Could you check a few things on this model? Use its own coordinates, in mm. A direction names the side the tool comes from. Coordinates: 2 decimals unless noted, no trailing zeros. Write each loop counter-clockwise with the first axis right and the second up, starting at its lowest first coordinate (ties: lowest second). Pieces come first, ordered by that corner, then holes.
Autodesk Inventor part; units mm, degrees
ref_plane "Work Plane1" through (0, 15, 0) normal (0, 1, 0) x (-1, 0, 0)
ref_plane "YZ Plane" through (0, 0, 0) normal (1, 0, 0) x (0, 1, 0)
ref_plane "XY Plane" through (0, 0, 0) normal (0, 0, 1) x (1, 0, 0)
sketch "Sketch1" plane through (0, 0, 0) normal (0, 0, 1) x (1, 0, 0)
  line L0 (37.75, -20.25) -> (-37.75, -20.25)
  line L1 (-37.75, -20.25) -> (-37.75, 20.25)
  line L2 (-37.75, 20.25) -> (37.75, 20.25)
  line L3 (37.75, 20.25) -> (37.75, -20.25)
  point P0 (0, 0)
  point P1 (0, 20.25)
  point P2 (37.75, 0)
  dimension "d0" = 40.5
  dimension "d1" = 75.5
extrude "Extrusion1" add sketch "Sketch1" along normal blind 3
sketch "Sketch2" plane through (-37.75, 20.25, 0) normal (0, 1, 0) x (1, 0, 0)
  point P0 (37.75, 0)
ref_plane "Work Plane1" through (0, 15, 0) normal (0, 1, 0) x (-1, 0, 0)
sketch "Sketch3" plane through (0, 15, 0) normal (0, 1, 0) x (-1, 0, 0)
  line L0 (-37.75, 3) -> (37.75, 3)
  line L1 (7.25, 3) -> (-7.25, 3)
  line L2 (-7.25, 3) -> (-7.25, 6)
  line L3 (-7.25, 6) -> (7.25, 6)
  line L4 (7.25, 6) -> (7.25, 3)
  line L5 (7.25, 3) -> (-7.25, 3)
  point P0 (0, 6)
  point P1 (0, 3)
  dimension "d20" = 14.5
  dimension "d21" = 3
extrude "Extrusion2" add sketch "Sketch3" along normal blind 10
sketch "Sketch4" plane through (0, 0, 3) normal (0, 0, 1) x (1, 0, 0)
  line L0 (-30, -7) -> (-5, -7)
  line L1 (-5, -7) -> (-5, -13)
  line L2 (-5, -13) -> (-30, -13)
  line L3 (-30, -13) -> (-30, -7)
  line L4 (37.75, 20.25) -> (-37.75, 20.25)
  line L5 (0, 20.25) -> (0, -20.25) construction
  line L6 (-37.75, -20.25) -> (37.75, -20.25)
  line L7 (30, -7) -> (5, -7)
  line L8 (5, -7) -> (5, -13)
  line L9 (5, -13) -> (30, -13)
  line L10 (30, -13) -> (30, -7)
  point P0 (0, 0)
  point P1 (-5, -10)
  point P2 (-17.5, -7)
  point P3 (7.25, 20.25)
  point P4 (-7.25, 20.25)
  point P5 (0, 0)
  dimension "d9" = 25
  dimension "d10" = 6
  dimension "d11" = 5
  dimension "d12" = 7
extrude "Extrusion3" add sketch "Sketch4" along normal blind 5
sketch "Sketch5" plane through (-30, -13, 3) normal (0, -1, 0) x (1, 0, 0)
  line L0 (25, 0) -> (0, 0)
  line L1 (5, 0) -> (20, 0)
  line L2 (20, 0) -> (20, 3.5)
  line L3 (20, 3.5) -> (5, 3.5)
  line L4 (5, 3.5) -> (5, 0)
  line L5 (35, 5) -> (60, 5)
  line L6 (0, 0) -> (0, 5)
  line L7 (0, 5) -> (25, 5)
  line L8 (30, -3) -> (30, 5) construction
  line L9 (55, 0) -> (40, 0)
  line L10 (40, 0) -> (40, 3.5)
  line L11 (40, 3.5) -> (55, 3.5)
  line L12 (55, 3.5) -> (55, 0)
  point P0 (47.5, 5)
  point P1 (0, 2.5)
  point P2 (12.5, 3.5)
  point P3 (12.5, 5)
  point P4 (47.5, 3.5)
  point P5 (20, 0)
  dimension "d15" = 15
  dimension "d16" = 3.5
extrude "Extrusion4" cut sketch "Sketch5" against normal blind 3
properties part number "Pomodoro Robot Torso's back"
1. If we mould it in two halves opening along X, with no side actions, what happens to faces 6 (the face through (0, 25, 5)), 7 (the face through (5, -10, 5)), 8 (the face through (-30, -10, 5))? For each: pulls with the +X half, pulls with the -X half, needs draft (parallel to the pull), parting line crosses it, or undercut.
Verdict:
face 6: needs draft
face 7: undercut
face 8: pulls with the -X half
2. On a 3-axis mill with a long thin cutter (end or side, diameter ignored), from which of +Z, -Z, +X, -X, +Y, -Y can I reach the whole of each face in a straight line? I mean faces 1 (the face through (30, -10, 5)), 2 (the face through (-17, -13, 7)), 3 (the face through (-5, -10, 5)), 4 (the face through (17, -10, 5)), 5 (the face through (0, 15, 5)). Say none if no direction works.
Verdict:
face 1: +Z, +X, +Y, -Y
face 2: +Z, +X, -X, -Y
face 3: +Z, -Y
face 4: -Y
face 5: +Z, +X, -X
3. I want a section at B-B on x = 14.5. Please give me the cut outline in (y, z), plus the area to 3 significant figures.
Verdict:
outline: (-20.25, 0) - (20.25, 0) - (20.25, 3) - (-7, 3) - (-7, 8) - (-13, 8) - (-13, 6.5) - (-10, 6.5) - (-10, 3) - (-20.25, 3) - close
area: 141 mm2
4. I want a section at C-C on z = 2. Please give me the cut outline in (x, y), plus the area to 3 significant figures.
Verdict:
outline: (-37.75, -20.25) - (37.75, -20.25) - (37.75, 20.25) - (-37.75, 20.25) - close
area: 3,060 mm2
5. For pin 1 (1 mm diameter, centred on x = 18.5, z = 4.5, fed in from -Y); pin 2 (2.5 mm diameter, centred on x = -15, z = 6, fed in from +Y); pin 3 (3.5 mm diameter, centred on x = -4.5, z = 1, fed in from +Y), each with a flat end and sliding along its axis, tell me the tip position at first contact or that it passes through.
Verdict:
pin 1: stops at y = -10
pin 2: stops at y = -7
pin 3: stops at y = 20.25
6. I want a section at D-D on y = 21.5. Please give me the cut outline in (x, z), plus the area to 3 significant figures.
Verdict:
outline: (-7.25, 3) - (7.25, 3) - (7.25, 6) - (-7.25, 6) - close
area: 43.5 mm2
7. I want a section at A-A on y = -12. Please give me the cut outline in (x, z).
Verdict:
outline: (-37.75, 0) - (37.75, 0) - (37.75, 3) - (30, 3) - (30, 8) - (5, 8) - (5, 3) - (-5, 3) - (-5, 8) - (-30, 8) - (-30, 3) - (-37.75, 3) - close; hole (-25, 3) - (-10, 3) - (-10, 6.5) - (-25, 6.5) - close; hole (10, 3) - (25, 3) - (25, 6.5) - (10, 6.5) - close
8. Please list where these lines run through material, in increasing order: line 1 along Z through (x, y) = (2, -6.5); line 2 along Y through (x, z) = (-24, 7.5); line 3 along X through (y, z) = (-9, 3.5).
Verdict:
line 1: z = 0 to 3
line 2: y = -13 to -7
line 3: x = -30 to -5, 5 to 30
